Source: CAD feature listing. Evaluate the final solid. Frame: model axes, mm. Face numbers are marked on the shaded views. A direction names the side the tool comes from. Give positions to 0.01 mm unless a question says otherwise; leave off trailing zeros. Write each loop counter-clockwise with the first axis right and the second up, starting at its lowest first coordinate (ties: lowest second). Pieces come first, ordered by that corner, then holes. Notation, with made-up numbers: M 5.25,89.25 L 46.25,89.25 A17 ccw 46.25,114.25 Z; hole C -2.75,-9 d2. An arc over 180 degrees is marked long. Return JSON: item names as keys, results as strings.
```python
from build123d import *

# Parameters (mm, degrees)
F0_W      = 700
F0_H      = 200
F1_DEPTH  = 400
F4_DEPTH  = 360
F5_R      = 15
F6_DEPTH  = 30
F7_W      = 60
F7_H      = 250
F8_DEPTH  = 60
F9_R      = 10
F10_DEPTH = 25


# Not quite as in the source:
# - a feature names something its author has since deleted; it is built from what else it names


with BuildPart() as f1:
    # F0 (on Front) → F1 (new body)
    with BuildSketch(Plane.XZ):
        with Locations((350, 100)):
            Rectangle(F0_W, F0_H)
    extrude(amount=-F1_DEPTH)

    # F3 (on offset) → F4 (join)
    with BuildSketch(Plane.XZ.offset(-20)):
        Polygon((20, -10), (20, -19.140496552), (20, -50), (20, -60), (30, -60), (80, -60), (80, -50), (30, -50), (30, -10), (80, -10), (80, 0), (20, 0), align=None)
        Polygon((680, -10), (680, 0), (620, 0), (620, -10), (670, -10), (670, -50), (620, -50), (620, -60), (670, -60), (680, -60), align=None)
    extrude(amount=-F4_DEPTH)

    # F5 (on face) → F6 (join)
    with BuildSketch(Plane.XZ):
        with BuildLine():
            ThreePointArc((48.0253212154, 139.9992847443), (37.4187194976, 135.6058864621), (33.0253212154, 124.9992847443))
            Line((33.0253212154, 124.9992847443), (48.0253212154, 124.9992847443))
            Line((48.0253212154, 124.9992847443), (48.0253212154, 139.9992847443))
        make_face()
        with BuildLine():
            ThreePointArc((648.0253212154, 124.9992847443), (633.0253212154, 139.9992847443), (618.0253212154, 124.9992847443))
            Line((618.0253212154, 124.9992847443), (648.0253212154, 124.9992847443))
        make_face()
        with BuildLine():
            Line((648.0253212154, 124.9992847443), (618.0253212154, 124.9992847443))
            ThreePointArc((618.0253212154, 124.9992847443), (633.0253212154, 109.9992847443), (648.0253212154, 124.9992847443))
        make_face()
        with BuildLine():
            ThreePointArc((583.0253212154, 124.9992847443), (568.0253212154, 139.9992847443), (553.0253212154, 124.9992847443))
            Line((553.0253212154, 124.9992847443), (583.0253212154, 124.9992847443))
        make_face()
        with BuildLine():
            Line((583.0253212154, 124.9992847443), (553.0253212154, 124.9992847443))
            ThreePointArc((553.0253212154, 124.9992847443), (568.0253212154, 109.9992847443), (583.0253212154, 124.9992847443))
        make_face()
        with BuildLine():
            ThreePointArc((518.0253212154, 124.9992847443), (503.0253212154, 139.9992847443), (488.0253212154, 124.9992847443))
            Line((488.0253212154, 124.9992847443), (518.0253212154, 124.9992847443))
        make_face()
        with BuildLine():
            Line((518.0253212154, 124.9992847443), (488.0253212154, 124.9992847443))
            ThreePointArc((488.0253212154, 124.9992847443), (503.0253212154, 109.9992847443), (518.0253212154, 124.9992847443))
        make_face()
        with BuildLine():
            ThreePointArc((453.0253212154, 124.9992847443), (438.0253212154, 139.9992847443), (423.0253212154, 124.9992847443))
            Line((423.0253212154, 124.9992847443), (453.0253212154, 124.9992847443))
        make_face()
        with BuildLine():
            Line((453.0253212154, 124.9992847443), (423.0253212154, 124.9992847443))
            ThreePointArc((423.0253212154, 124.9992847443), (438.0253212154, 109.9992847443), (453.0253212154, 124.9992847443))
        make_face()
        with BuildLine():
            ThreePointArc((388.0253212154, 124.9992847443), (373.0253212154, 139.9992847443), (358.0253212154, 124.9992847443))
            Line((358.0253212154, 124.9992847443), (388.0253212154, 124.9992847443))
        make_face()
        with BuildLine():
            Line((388.0253212154, 124.9992847443), (358.0253212154, 124.9992847443))
            ThreePointArc((358.0253212154, 124.9992847443), (373.0253212154, 109.9992847443), (388.0253212154, 124.9992847443))
        make_face()
        with BuildLine():
            ThreePointArc((323.0253212154, 124.9992847443), (308.0253212154, 139.9992847443), (293.0253212154, 124.9992847443))
            Line((293.0253212154, 124.9992847443), (323.0253212154, 124.9992847443))
        make_face()
        with BuildLine():
            Line((323.0253212154, 124.9992847443), (293.0253212154, 124.9992847443))
            ThreePointArc((293.0253212154, 124.9992847443), (308.0253212154, 109.9992847443), (323.0253212154, 124.9992847443))
        make_face()
        with BuildLine():
            ThreePointArc((258.0253212154, 124.9992847443), (243.0253212154, 139.9992847443), (228.0253212154, 124.9992847443))
            Line((228.0253212154, 124.9992847443), (258.0253212154, 124.9992847443))
        make_face()
        with BuildLine():
            Line((258.0253212154, 124.9992847443), (228.0253212154, 124.9992847443))
            ThreePointArc((228.0253212154, 124.9992847443), (243.0253212154, 109.9992847443), (258.0253212154, 124.9992847443))
        make_face()
        with BuildLine():
            ThreePointArc((193.0253212154, 124.9992847443), (178.0253212154, 139.9992847443), (163.0253212154, 124.9992847443))
            Line((163.0253212154, 124.9992847443), (193.0253212154, 124.9992847443))
        make_face()
        with BuildLine():
            Line((193.0253212154, 124.9992847443), (163.0253212154, 124.9992847443))
            ThreePointArc((163.0253212154, 124.9992847443), (178.0253212154, 109.9992847443), (193.0253212154, 124.9992847443))
        make_face()
        with BuildLine():
            ThreePointArc((128.0253212154, 124.9992847443), (113.0253212154, 139.9992847443), (98.0253212154, 124.9992847443))
            Line((98.0253212154, 124.9992847443), (128.0253212154, 124.9992847443))
        make_face()
        with BuildLine():
            Line((128.0253212154, 124.9992847443), (98.0253212154, 124.9992847443))
            ThreePointArc((98.0253212154, 124.9992847443), (113.0253212154, 109.9992847443), (128.0253212154, 124.9992847443))
        make_face()
        with BuildLine():
            ThreePointArc((63.0253212154, 74.9992847443), (58.6319229332, 85.6058864621), (48.0253212154, 89.9992847443))
            Line((48.0253212154, 89.9992847443), (48.0253212154, 59.9992847443))
            ThreePointArc((48.0253212154, 59.9992847443), (58.6319229332, 64.3926830265), (63.0253212154, 74.9992847443))
        make_face()
        with BuildLine():
            Line((48.0253212154, 59.9992847443), (48.0253212154, 89.9992847443))
            ThreePointArc((48.0253212154, 89.9992847443), (33.0253212154, 74.9992847443), (48.0253212154, 59.9992847443))
        make_face()
        with BuildLine():
            Line((48.0253212154, 124.9992847443), (33.0253212154, 124.9992847443))
            ThreePointArc((33.0253212154, 124.9992847443), (37.4187194976, 114.3926830265), (48.0253212154, 109.9992847443))
            Line((48.0253212154, 109.9992847443), (48.0253212154, 124.9992847443))
        make_face()
        with BuildLine():
            Line((48.0253212154, 139.9992847443), (48.0253212154, 124.9992847443))
            Line((48.0253212154, 124.9992847443), (63.0253212154, 124.9992847443))
            ThreePointArc((63.0253212154, 124.9992847443), (58.6319229332, 135.6058864621), (48.0253212154, 139.9992847443))
        make_face()
        with BuildLine():
            Line((63.0253212154, 124.9992847443), (48.0253212154, 124.9992847443))
            Line((48.0253212154, 124.9992847443), (48.0253212154, 109.9992847443))
            ThreePointArc((48.0253212154, 109.9992847443), (58.6319229332, 114.3926830265), (63.0253212154, 124.9992847443))
        make_face()
        with Locations((113.0253212154, 74.9992847443)):
            Circle(F5_R)
        with Locations((178.0253212154, 74.9992847443)):
            Circle(F5_R)
        with Locations((243.0253212154, 74.9992847443)):
            Circle(F5_R)
        with Locations((308.0253212154, 74.9992847443)):
            Circle(F5_R)
        with Locations((373.0253212154, 74.9992847443)):
            Circle(F5_R)
        with Locations((438.0253212154, 74.9992847443)):
            Circle(F5_R)
        with Locations((503.0253212154, 74.9992847443)):
            Circle(F5_R)
        with Locations((568.0253212154, 74.9992847443)):
            Circle(F5_R)
        with Locations((633.0253212154, 74.9992847443)):
            Circle(F5_R)
    extrude(amount=F6_DEPTH)

    # F7 (on face) → F8 (join)
    with BuildSketch(Plane.XY.offset(200)):
        with Locations((81.3367652893, 190.7173022628)):
            Rectangle(F7_W, F7_H)
        with Locations((151.3367652893, 190.7173022628)):
            Rectangle(F7_W, F7_H)
        with Locations((221.3367652893, 190.7173022628)):
            Rectangle(F7_W, F7_H)
        with Locations((291.3367652893, 190.7173022628)):
            Rectangle(F7_W, F7_H)
        with Locations((361.3367652893, 190.7173022628)):
            Rectangle(F7_W, F7_H)
        with Locations((431.3367652893, 190.7173022628)):
            Rectangle(F7_W, F7_H)
        with Locations((501.3367652893, 190.7173022628)):
            Rectangle(F7_W, F7_H)
        with Locations((571.3367652893, 190.7173022628)):
            Rectangle(F7_W, F7_H)
        with Locations((641.3367652893, 190.7173022628)):
            Rectangle(F7_W, F7_H)
    extrude(amount=F8_DEPTH)

    # F9 (on face) → F10 (cut)
    with BuildSketch(Plane(origin=(0, 0, -60), x_dir=(1, 0, 0), z_dir=(0, 0, -1))):
        with BuildLine():
            ThreePointArc((50, -310), (40, -320), (50, -330))
            Line((50, -330), (50, -310))
        make_face()
        with BuildLine():
            ThreePointArc((50, -70), (40, -80), (50, -90))
            Line((50, -90), (50, -70))
        make_face()
        with BuildLine():
            Line((50, -70), (50, -90))
            ThreePointArc((50, -90), (57.0710678119, -87.0710678119), (60, -80))
            ThreePointArc((60, -80), (57.0710678119, -72.9289321881), (50, -70))
        make_face()
        with BuildLine():
            Line((50, -310), (50, -330))
            ThreePointArc((50, -330), (57.0710678119, -327.0710678119), (60, -320))
            ThreePointArc((60, -320), (57.0710678119, -312.9289321881), (50, -310))
        make_face()
        with Locations((650.3430891037, -320)):
            Circle(F9_R)
        with Locations((650.3430891037, -80)):
            Circle(F9_R)
    extrude(amount=-F10_DEPTH, mode=Mode.SUBTRACT)


solid = f1.part
```
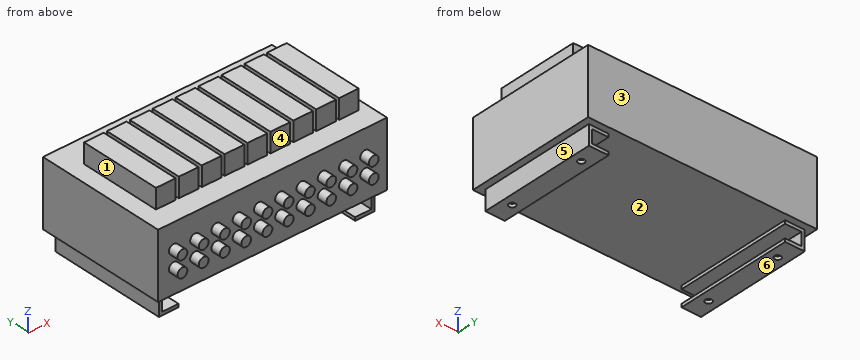
1) Line query: line 1 (X direction, y = 80, z = -52); line 2 (Z direction, x = 44, y = 35); line 3 (X direction, y = 338.5, z = -14.5). Output: solid intervals per line, ascending. Write a range as [from, to].
Numbers:
{"line 1": "x = [20, 40], [60, 80], [620, 640.34], [660.34, 680]", "line 2": "z = [-60, -50], [-10, 200]", "line 3": "x = [20, 30], [670, 680]"}
2) Cut plane B-B, the plane y = 50. Return the cut outline in (x, z).
Numbers:
{"outline": "M 0,0 L 20,0 L 20,-60 L 80,-60 L 80,-50 L 30,-50 L 30,-10 L 80,-10 L 80,0 L 620,0 L 620,-10 L 670,-10 L 670,-50 L 620,-50 L 620,-60 L 680,-60 L 680,0 L 700,0 L 700,200 L 0,200 Z"}
3) Contact query for flat-ended pins moving along their axis: pin 1 Ø2 at (x, y) = (226.5, 321) entering from +Z; pin 2 Ø18 at (y, z) = (184.5, 240) entering from -X; pin 3 Ø18 at (x, z) = (77.5, 240) entering from -Y. Output: stop coordinate, or through.
Numbers:
{"pin 1": "stops at z = 200", "pin 2": "stops at x = 51.34", "pin 3": "stops at y = 65.72"}
4) Cut plane C-C, the plane x = 438. Return the cut outline in (y, z), then the cut area to 3 significant figures.
Numbers:
{"outline": "M -30,60 L 0,60 L 0,0 L 400,0 L 400,200 L 315.72,200 L 315.72,260 L 65.72,260 L 65.72,200 L 0,200 L 0,140 L -30,140 L -30,110 L 0,110 L 0,90 L -30,90 Z", "area": "96,800 mm²"}
5) Set-up query: the marked faces 4, 5 and 6. Return all of +Z, -Z, +X, -X, +Y, -Y with unobstructed straight access to the full face (end or side cutting, diameter ignored); none if empty.
Numbers:
{"face 4": "+Z, +X, -X, -Y", "face 5": "-Z, +X, +Y, -Y", "face 6": "-Z, +X, -X, +Y, -Y"}
6) Cut plane A-A, the plane x = 591. Return the cut outline in (y, z), then the cut area to 3 significant figures.
Numbers:
{"outline": "M 0,0 L 400,0 L 400,200 L 315.72,200 L 315.72,260 L 65.72,260 L 65.72,200 L 0,200 Z", "area": "95,000 mm²"}
7) Draft query along X for the marked faces 1, 2 and 3. Return one class per face: released by +X, released by -X, zero draft, split by the parting line, or undercut.
Numbers:
{"face 1": "released by -X", "face 2": "undercut", "face 3": "zero draft"}
